```python
from build123d import *

# Parameters (mm, degrees)
BOSS_EXTRUDE1_DEPTH      = 2
BOSS_EXTRUDE1_DEPTH_BACK = 7
BOSS_EXTRUDE3_DEPTH      = 9
SKETCH6_R                = 4
CUT_EXTRUDE1_DEPTH       = 18
BOSS_EXTRUDE4_DEPTH      = 18
SKETCH8_R                = 2.25
CUT_EXTRUDE2_DEPTH       = 69.863255609
CUT_EXTRUDE3_DEPTH       = 67.431528446
CUT_EXTRUDE3_DEPTH_BACK  = 67.431528446
SKETCH9_W                = 10.323299019
SKETCH9_H                = 27.481333942
SKETCH10_W               = 25.230248524
SKETCH10_H               = 17.693033904
CUT_EXTRUDE4_DEPTH       = 67.436499079


with BuildPart() as part:
    # Sketch2 → Boss-Extrude1 (new, two sides: drawn at the far end of the back side and taken through both)
    with BuildSketch(Plane.XY.offset(-BOSS_EXTRUDE1_DEPTH_BACK)):
        with BuildLine():
            Line((17.593003447, 3.447921134), (18.432689254, 3.812129579))
            ThreePointArc((18.432689254, 3.812129579), (18.142308848, 4.822341152), (17.760116965, 5.801513031))
            Line((17.760116965, 5.801513031), (16.871688472, 5.581479263))
            Line((16.871688472, 5.581479263), (15.649099733, 5.241598415))
            ThreePointArc((15.649099733, 5.241598415), (15.22663553, 6.009376293), (14.733410626, 6.733729845))
            Line((14.733410626, 6.733729845), (15.590096731, 7.669855443))
            Line((15.590096731, 7.669855443), (16.188603379, 8.362321932))
            ThreePointArc((16.188603379, 8.362321932), (15.488665299, 9.146499772), (14.719475556, 9.862876308))
            Line((14.719475556, 9.862876308), (14.014498216, 9.279158058))
            Line((14.014498216, 9.279158058), (13.060452596, 8.442474621))
            ThreePointArc((13.060452596, 8.442474621), (12.346699165, 8.950918239), (11.588033655, 9.389535972))
            Line((11.588033655, 9.389535972), (11.95371149, 10.604658163))
            Line((11.95371149, 10.604658163), (12.192497398, 11.488231214))
            ThreePointArc((12.192497398, 11.488231214), (11.221632964, 11.891059284), (10.217792822, 12.202753318))
            Line((10.217792822, 12.202753318), (9.835896044, 11.370963143))
            Line((9.835896044, 11.370963143), (9.33935398, 10.203192533))
            ThreePointArc((9.33935398, 10.203192533), (8.475678941, 10.351598396), (7.601835833, 10.417606691))
            Line((7.601835833, 10.417606691), (7.404078418, 11.671055622))
            Line((7.404078418, 11.671055622), (7.235849109, 12.570732756))
            ThreePointArc((7.235849109, 12.570732756), (6.18634993, 12.512426015), (5.14668224, 12.357702722))
            Line((5.14668224, 12.357702722), (5.163505363, 11.442586867))
            Line((5.163505363, 11.442586867), (5.222813101, 10.175020376))
            ThreePointArc((5.222813101, 10.175020376), (4.380277888, 9.933994883), (3.564332526, 9.614319987))
            Line((3.564332526, 9.614319987), (2.842308143, 10.657834724))
            Line((2.842308143, 10.657834724), (2.300383494, 11.395423851))
            ThreePointArc((2.300383494, 11.395423851), (1.380115753, 10.887530665), (0.510539453, 10.297034891))
            Line((0.510539453, 10.297034891), (0.922750452, 9.479843274))
            Line((0.922750452, 9.479843274), (1.526161366, 8.363537991))
            ThreePointArc((1.526161366, 8.363537991), (0.871640411, 7.780819197), (0.275200782, 7.138776643))
            Line((0.275200782, 7.138776643), (-0.828084785, 7.765676295))
            Line((-0.828084785, 7.765676295), (-1.636369952, 8.195088843))
            ThreePointArc((-1.636369952, 8.195088843), (-2.245135941, 7.338203686), (-2.772390602, 6.42889036))
            Line((-2.772390602, 6.42889036), (-2.04643517, 5.871477804))
            Line((-2.04643517, 5.871477804), (-1.018434012, 5.12753168))
            ThreePointArc((-1.018434012, 5.12753168), (-1.355304806, 4.318534189), (-1.61410652, 3.481288379))
            Line((-1.61410652, 3.481288379), (-2.880134034, 3.567407782))
            Line((-2.880134034, 3.567407782), (-3.794688927, 3.603593329))
            ThreePointArc((-3.794688927, 3.603593329), (-3.971379595, 2.567432815), (-4.051883364, 1.519402593))
            Line((-4.051883364, 1.519402593), (-3.155967876, 1.332171491))
            Line((-3.155967876, 1.332171491), (-1.90698471, 1.107932181))
            ThreePointArc((-1.90698471, 1.107932181), (-1.859483953, 0.232887867), (-1.729388897, -0.633734398))
            Line((-1.729388897, -0.633734398), (-2.907406081, -1.105452248))
            Line((-2.907406081, -1.105452248), (-3.747091888, -1.469660694))
            ThreePointArc((-3.747091888, -1.469660694), (-3.456711482, -2.479872267), (-3.0745196, -3.459044145))
            Line((-3.0745196, -3.459044145), (-2.186091107, -3.239010378))
            Line((-2.186091107, -3.239010378), (-0.963502367, -2.899129529))
            ThreePointArc((-0.963502367, -2.899129529), (-0.541038164, -3.666907408), (-0.047813261, -4.391260959))
            Line((-0.047813261, -4.391260959), (-0.904499365, -5.327386558))
            Line((-0.904499365, -5.327386558), (-1.503006014, -6.019853046))
            ThreePointArc((-1.503006014, -6.019853046), (-0.803067933, -6.804030887), (-0.03387819, -7.520407423))
            Line((-0.03387819, -7.520407423), (0.67109915, -6.936689172))
            Line((0.67109915, -6.936689172), (1.625144769, -6.100005735))
            ThreePointArc((1.625144769, -6.100005735), (2.3388982, -6.608449353), (3.097563711, -7.047067087))
            Line((3.097563711, -7.047067087), (2.731885876, -8.262189278))
            Line((2.731885876, -8.262189278), (2.493099968, -9.145762328))
            ThreePointArc((2.493099968, -9.145762328), (3.463964401, -9.548590398), (4.467804544, -9.860284433))
            Line((4.467804544, -9.860284433), (4.849701322, -9.028494257))
            Line((4.849701322, -9.028494257), (5.346243386, -7.860723648))
            ThreePointArc((5.346243386, -7.860723648), (6.209918425, -8.009129511), (7.083761533, -8.075137806))
            Line((7.083761533, -8.075137806), (7.281518948, -9.328586736))
            Line((7.281518948, -9.328586736), (7.449748257, -10.22826387))
            ThreePointArc((7.449748257, -10.22826387), (8.499247436, -10.16995713), (9.538915126, -10.015233837))
            Line((9.538915126, -10.015233837), (9.522092003, -9.100117982))
            Line((9.522092003, -9.100117982), (9.462784265, -7.83255149))
            ThreePointArc((9.462784265, -7.83255149), (10.305319478, -7.591525998), (11.12126484, -7.271851101))
            Line((11.12126484, -7.271851101), (11.843289223, -8.315365839))
            Line((11.843289223, -8.315365839), (12.385213872, -9.052954966))
            ThreePointArc((12.385213872, -9.052954966), (13.305481612, -8.54506178), (14.175057913, -7.954566005))
            Line((14.175057913, -7.954566005), (13.762846914, -7.137374389))
            Line((13.762846914, -7.137374389), (13.159436, -6.021069105))
            ThreePointArc((13.159436, -6.021069105), (13.813956955, -5.438350311), (14.410396584, -4.796307757))
            Line((14.410396584, -4.796307757), (15.513682151, -5.42320741))
            Line((15.513682151, -5.42320741), (16.321967317, -5.852619957))
            ThreePointArc((16.321967317, -5.852619957), (16.930733307, -4.9957348), (17.457987967, -4.086421474))
            Line((17.457987967, -4.086421474), (16.732032536, -3.529008918))
            Line((16.732032536, -3.529008918), (15.704031377, -2.785062794))
            ThreePointArc((15.704031377, -2.785062794), (16.040902172, -1.976065303), (16.299703886, -1.138819493))
            Line((16.299703886, -1.138819493), (17.565731399, -1.224938896))
            Line((17.565731399, -1.224938896), (18.480286292, -1.261124443))
            ThreePointArc((18.480286292, -1.261124443), (18.656976961, -0.22496393), (18.737480729, 0.823066292))
            Line((18.737480729, 0.823066292), (17.841565242, 1.010297394))
            Line((17.841565242, 1.010297394), (16.592582076, 1.234536705))
            ThreePointArc((16.592582076, 1.234536705), (16.545081318, 2.109581019), (16.414986263, 2.976203284))
            Line((16.414986263, 2.976203284), (17.593003447, 3.447921134))
        make_face()
    extrude(amount=BOSS_EXTRUDE1_DEPTH + BOSS_EXTRUDE1_DEPTH_BACK)

    # Sketch5 → Boss-Extrude3 (add)
    with BuildSketch(Plane.XY.offset(2)):
        with BuildLine():
            Line((34.627961915, -50.407866333), (38.369192873, -48.55177457))
            Line((38.369192873, -48.55177457), (13.393984011, -14.920355903))
            Line((13.393984011, -14.920355903), (9.462784265, -7.83255149))
            Line((9.462784265, -7.83255149), (0.865656202, -2.843190202))
            Line((0.865656202, -2.843190202), (-0.03387819, -7.520407423))
            add(Edge.make_bspline(
                [(34.627961915, -50.407866333), (20.737528927, -38.343464696), (7.957182105, -24.264537371), (-0.03387819, -7.520407423)],
                knots=[0, 0, 0, 0, 1, 1, 1, 1], degree=3))
        make_face()
    extrude(amount=-BOSS_EXTRUDE3_DEPTH)

    # Sketch6 → Cut-Extrude1 (cut)
    with BuildSketch(Plane(origin=(0, 0, -7), x_dir=(-1, 0, 0), z_dir=(0, 0, -1))):
        with Locations((-7.342798683, 1.171234443)):
            Circle(SKETCH6_R)
    extrude(amount=-CUT_EXTRUDE1_DEPTH, mode=Mode.SUBTRACT)

    # Sketch7 → Boss-Extrude4 (add)
    with BuildSketch(Plane.XY.offset(2)):
        with BuildLine():
            Line((34.627961915, -50.407866333), (38.369192873, -48.55177457))
            Line((38.369192873, -48.55177457), (13.393984011, -14.920355903))
            add(Edge.make_bspline(
                [(7.977955023, -21.345123668), (8.112113434, -15.921271934), (13.393984011, -14.920355903)],
                knots=[0, 0, 0, 1, 1, 1], degree=2))
            add(Edge.make_bspline(
                [(7.977955023, -21.345123668), (15.413845314, -32.210109704), (24.739621619, -41.819443715), (34.627961915, -50.407866333)],
                knots=[0.288118642, 0.288118642, 0.288118642, 0.288118642, 1, 1, 1, 1], degree=3))
        make_face()
    extrude(amount=BOSS_EXTRUDE4_DEPTH)

    # Sketch8 → Cut-Extrude2 (cut, through all)
    with BuildSketch(Plane(origin=(0, 0, -7), x_dir=(-1, 0, 0), z_dir=(0, 0, -1))):
        with Locations((-14.312794722, -23.020807584)):
            Circle(SKETCH8_R)
        with Locations((-25.785580409, -37.215397344)):
            Circle(SKETCH8_R)
    extrude(amount=-CUT_EXTRUDE2_DEPTH, mode=Mode.SUBTRACT)

    # Sketch9 → Cut-Extrude3 (cut, two sides: drawn at the far end of the back side and taken through both)
    with BuildSketch(Plane(origin=(0, 0, 0), x_dir=(0, 0, -1), z_dir=(1, 0, 0)).offset(-CUT_EXTRUDE3_DEPTH_BACK)):
        with Locations((-4.16164951, 3.801629666)):
            Rectangle(SKETCH9_W, SKETCH9_H)
    extrude(amount=CUT_EXTRUDE3_DEPTH + CUT_EXTRUDE3_DEPTH_BACK, mode=Mode.SUBTRACT)

    # Sketch10 → Cut-Extrude4 (cut, through all)
    with BuildSketch(Plane(origin=(1.491415785, 1.107548305, 0), x_dir=(0, 0, -1), z_dir=(0.8028367498889462, 0.5961989206865052, 0))):
        with Locations((-14.573721534, -16.286562524)):
            Rectangle(SKETCH10_W, SKETCH10_H)
    extrude(amount=-CUT_EXTRUDE4_DEPTH, mode=Mode.SUBTRACT)


solid = part.part
```
Check sheet for the modelled part. Datum: model origin and axes. Units: mm. A direction names the side the tool comes from. Coordinates: 2 decimals unless noted, no trailing zeros. Write each loop counter-clockwise with the first axis right and the second up, starting at its lowest first coordinate (ties: lowest second). Pieces come first, ordered by that corner, then holes. Notation, with made-up numbers: M 12,10 L 58,10 A19 cw 58,42 Z; hole C -20.75,0.5 d7. An arc over 180 degrees is marked long. Write item = value, one per line. Start each with the question number.
1. Go/stop test with flat-tipped pins: pin 1 (2 mm diameter, centred on y = -35, z = 3, fed in from -X); pin 2 (3.5 mm diameter, centred on x = 5, z = 1, fed in from +Y); pin 3 (1.5 mm diameter, centred on y = -42, z = 12.5, fed in from -X); pin 4 (4 mm diameter, centred on x = 19, y = -5.5, fed in from -Z). Record where each tip stops, or that it passes through.
2. Mould release check, pull along Y, two halves, no side actions. Record for faces 1 (the flat face through (7, -4, -1)), 2 (the cylindrical face through (-2.237, 7.351, -4.042)), 3 (the cylindrical face through (-1.86, 0.25, -4.04)): pulls with the +Y half, pulls with the -Y half, needs draft (parallel to the pull), parting line crosses it, or undercut.
3. Tool access check on faces 4 (the cylindrical face through (-3.46, -2.47, -4.04)), 5 (the flat face through (11, -11, 2)), 6 (the flat face through (-2.54, 1.22, -4.04)), 7 (the cylindrical face through (0.88, 7.79, -4.04)). Record the directions out of +Z, -Z, +X, -X, +Y, -Y that give a thin tool (end or side, any length) a straight path to the whole face; none if there is none.
4. Thickness scan on probe 1 along Y at (x, z) = (17.5, -4.5); probe 2 along Z at (x, y) = (7, -10.5); probe 3 along Y at (x, z) = (25.5, 11.5). Record the ranges inside material, lowest first.
5. Sectioned sample at B-B (z = 0.25). State how many separate pieces and enclosed holes the cut face has, then the cut area to 3 significant figures.
6. Sectioned sample at A-A (x = 36.5). Record the cut outline in (y, z).
The answers:
q1.pin_1 = 17.9
q1.pin_2 = -9.94
q1.pin_3 = 24.75
q1.pin_4 = through
q2.face_1 = needs draft
q2.face_2 = pulls with the +Y half
q2.face_3 = undercut
q3.face_4 = +Z, -Z, -X, -Y
q3.face_5 = +Z, +X, -X, +Y
q3.face_6 = +Z, -Z, -X
q3.face_7 = +Z, -Z
q4.probe_1 = -33.54 to -20.45, -1.22 to 1.07, 3.41 to 5.74
q4.probe_2 = -7 to 1.96
q4.probe_3 = -41.99 to -39.45, -34.98 to -31.22
q5.separate_pieces = 1
q5.enclosed_holes = 2
q5.area = 330 mm²
q6.outline = M -49.48,-7 L -46.03,-7 L -46.03,20 L -49.48,20 Z
